Part model, mm, in its own coordinate system. A direction names the side the tool comes from. Give positions to 0.01 mm unless a question says otherwise; leave off trailing zeros. Write each loop counter-clockwise with the first axis right and the second up, starting at its lowest first coordinate (ties: lowest second). Pieces come first, ordered by that corner, then holes.
Autodesk Inventor part; units mm, degrees
ref_plane "YZ Plane" through (0, 0, 0) normal (1, 0, 0) x (0, 1, 0)
ref_plane "XZ Plane" through (0, 0, 0) normal (0, 1, 0) x (-1, 0, 0)
ref_plane "XY Plane" through (0, 0, 0) normal (0, 0, 1) x (1, 0, 0)
sketch "Sketch1" plane through (0, 0, 0) normal (0, 0, 1) x (1, 0, 0)
  line L0 (-10.014, 0) -> (-10.014, 3)
  line L1 (-10.014, 3) -> (39.986, 3)
  line L2 (39.986, 3) -> (39.986, 3.5)
  line L3 (41.486, 5) -> (66.986, 5)
  line L4 (69.986, 2) -> (69.986, 0)
  arc A0 (41.486, 5) -> (39.986, 3.5) centre (41.486, 3.5) ccw
  arc A1 (69.986, 2) -> (66.986, 5) centre (66.986, 2) ccw
  line L5 (-10.014, 0) -> (69.986, 0)
  point P0 (0, 0)
  point P1 (39.986, 5)
  point P2 (69.986, 5)
  dimension "d0" = 3
  dimension "d1" = 50
  dimension "d2" = 2
  dimension "d3" = 30
  dimension "d4" = 1.5
  dimension "d5" = 3
revolve "Revolution1" add sketch "Sketch1" angle 360 about axis through (-10.014, 0, 0) along (1, 0, 0)
properties part number "ocas" material "Wood (Birch)"
1) 3-axis set-ups, long thin cutter, end or side, ignore diameter. For faces 1 (the face through (69.986, 0, 0)), 2 (the face through (39.986, 3, 1)): which of +Z, -Z, +X, -X, +Y, -Y reach the whole face in a straight line?
Answers follow:
face 1: +Z, -Z, +X, +Y, -Y
face 2: -X
2) Wall check: L1, parallel to Z at x = 9, y = -2.25; L2, parallel to Z at x = 65.5, y = 0.25; L3, parallel to Y at x = 45, z = 4. Give the ranges that are in metal, low to high.
Answers follow:
L1: z = -1.98 to 1.98
L2: z = -4.99 to 4.99
L3: y = -3 to 3
3) Saw through at A-A, the plane x = 3. Write the cut outline in (y, z), then the cut area to 3 significant figures.
Answers follow:
outline: circle Ø6 at (0, 0)
area: 28.3 mm2
4) Pin check, flat tips, straight feed: pin 1 Ø1 at (x, z) = (19.5, 0.5) entering from +Y; pin 2 Ø3 at (x, z) = (51, -3.5) entering from +Y; pin 3 Ø2 at (x, y) = (52, -2.5) entering from -Z. Stop position of each tip, or through.
Answers follow:
pin 1: stops at y = 3
pin 2: stops at y = 4.58
pin 3: stops at z = -4.77
